Geometry: final body of the model. Coordinates: model frame, mm. Face numbers are marked on the shaded views. A direction names the side the tool comes from. Round coordinates to 2 decimals unless told otherwise and drop trailing zeros. Write each loop counter-clockwise with the first axis right and the second up, starting at its lowest first coordinate (ties: lowest second). Pieces come first, ordered by that corner, then holes. Notation, with made-up numbers: (14, 30) - (46, 30) arc R23 cw to (46, 38) - close; hole circle Ø11 at (-19.5, 5.5). An arc over 180 degrees is marked (long way). Write each question's results on one line, items separated by ' | '.
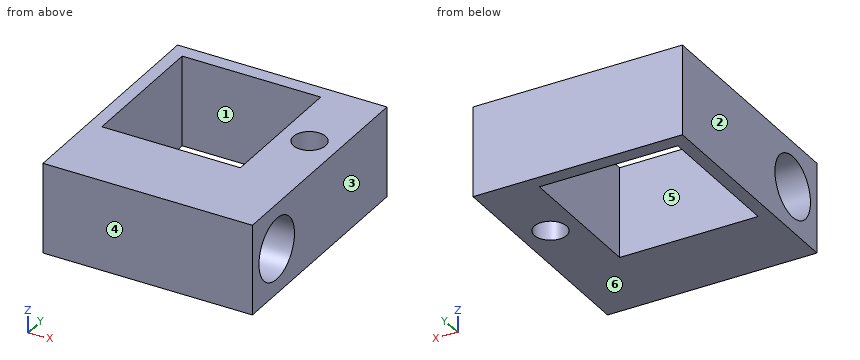
from build123d import *

# Parameters (mm, degrees)
SKETCH1_W           = 65
SKETCH1_H           = 72
SKETCH1_R           = 5
SKETCH1_W_2         = 43
SKETCH1_H_2         = 43
BOSS_EXTRUDE1_DEPTH = 28
SKETCH2_R           = 9.5
CUT_EXTRUDE1_DEPTH  = 80.404030124


with BuildPart() as part:
    # Sketch1 → Boss-Extrude1 (new body)
    with BuildSketch(Plane.XY):
        Rectangle(SKETCH1_W, SKETCH1_H)
        with Locations((23.5, 10.069230769)):
            Circle(SKETCH1_R, mode=Mode.SUBTRACT)
        with Locations((-7, 10.069230769)):
            Rectangle(SKETCH1_W_2, SKETCH1_H_2, mode=Mode.SUBTRACT)
    extrude(amount=BOSS_EXTRUDE1_DEPTH)

    # Sketch2 → Cut-Extrude1 (cut, through all)
    with BuildSketch(Plane(origin=(32.5, 0, 0), x_dir=(0, 0, -1), z_dir=(1, 0, 0))):
        with Locations((-14, -23)):
            Circle(SKETCH2_R)
    extrude(amount=-CUT_EXTRUDE1_DEPTH, mode=Mode.SUBTRACT)


solid = part.part
Q1. Ray query, line 1 along Y through (x, z) = (11.5, 14); line 2 along X through (y, z) = (19, 1.5); line 3 along X through (y, z) = (13, 20). Return the intervals inside material, ascending.
Answer block:
line 1: -36 to -32.5, -13.5 to -11.43, 31.57 to 36 | line 2: -32.5 to -28.5, 14.5 to 32.5 | line 3: -32.5 to -28.5, 14.5 to 19.45, 27.55 to 32.5
Q2. Section query B-B, the plane y = -23. Return loops of the section in (x, z), plus the area to 3 significant figures.
Answer block:
outline: (-32.5, 0) - (32.5, 0) - (32.5, 4.5) - (-32.5, 4.5) - close; (-32.5, 23.5) - (32.5, 23.5) - (32.5, 28) - (-32.5, 28) - close | area: 585 mm2
Q3. Access query for the marked faces 5 and 6. Directions: +Z, -Z, +X, -X, +Y, -Y. A direction counts if a zero-diameter tool reaches every point of the face in a straight line with its end or side. Return the directions, or none.
Answer block:
face 5: +Z, -Z | face 6: -Z, +X, -X, +Y, -Y
Q4. Section query A-A, the plane x = -20. Return loops of the section in (y, z).
Answer block:
outline: (-36, 0) - (-11.43, 0) - (-11.43, 28) - (-36, 28) - close; (31.57, 0) - (36, 0) - (36, 28) - (31.57, 28) - close; hole circle Ø19 at (-23, 14)
Q5. Section query D-D, the plane x = 23.5. Return loops of the section in (y, z).
Answer block:
outline: (-36, 0) - (5.07, 0) - (5.07, 28) - (-36, 28) - close; (15.07, 0) - (36, 0) - (36, 28) - (15.07, 28) - close; hole circle Ø19 at (-23, 14)
Q6. Mould query, pull axis X, two halves, no side actions, for the marked faces 1, 2, 3 and 4. Classes: pulls with the +X half, pulls with the -X half, needs draft (parallel to the pull), parting line crosses it, or undercut.
Answer block:
face 1: undercut | face 2: pulls with the -X half | face 3: pulls with the +X half | face 4: needs draft
Q7. Section query C-C, the plane z = 14. Return loops of the section in (x, y), plus the area to 3 significant figures.
Answer block:
outline: (-32.5, -36) - (32.5, -36) - (32.5, -32.5) - (-32.5, -32.5) - close; (-32.5, -13.5) - (32.5, -13.5) - (32.5, 36) - (-32.5, 36) - close; hole (-28.5, -11.43) - (14.5, -11.43) - (14.5, 31.57) - (-28.5, 31.57) - close; hole circle Ø10 at (23.5, 10.07) | area: 1,520 mm2
